Verification items for the finished model (mm, model axes). Face numbers are marked on the shaded views. Give positions to 0.01 mm unless a question says otherwise; leave off trailing zeros. Order: outer loops, then holes, each group sorted by start corner. A loop starts at its lowest first (then second) coordinate and runs counter-clockwise, first axis right, second up. Notation, with made-up numbers: (34.5, 59.25) - (47.5, 59.25) arc R27 cw to (47.5, 87.25) - close; hole circle Ø1 at (-0.5, 12). An arc over 180 degrees is marked (long way). Answer as a JSON object with one key per item and string values. Group by question number.
(1) Mould release check, pull along X, two halves, no side actions. Record for the marked faces 1, 2 and 3: +X half, -X half, draft (parallel to the pull), parting line (faces both ways), or undercut.
(2) Thickness scan on line 1 (X direction, y = 18, z = -4); line 2 (Y direction, x = 8.25, z = -1.5); line 3 (Z direction, x = 13, y = 52.5). Record the ranges inside material, lowest first.
(3) Section check B-B (x = 4). Record the boundary of the cut face in (y, z).
(4) Section check A-A (z = -4). Record the boundary of the cut face in (x, y).
(5) Depth check by flat-ended pin: pin 1 Ø12 at (x, y) = (11, 56.5) entering from +Z; pin 2 Ø10 at (x, y) = (4, 55.5) entering from -Z; pin 3 Ø5 at (x, z) = (26, -4) entering from +Y; pin 4 Ø3.5 at (x, z) = (4, -26) entering from -Y. Enter the tip coordinate at first touch or a pass-through.
(6) Section check C-C (y = 9). Record the boundary of the cut face in (x, z), then the cut area to 3 significant figures.
(7) Section check D-D (z = -15). Record the boundary of the cut face in (x, y), then the cut area to 3 significant figures.
```python
from build123d import *

# Parameters (mm, degrees)
IZIM1_W                     = 30
IZIM1_H                     = 30
Y_KSEKLIK_EKSTR_ZYON1_DEPTH = 40
IZIM2_R                     = 2
KES_EKSTR_ZYON1_DEPTH       = 40
IZIM3_R                     = 10
IZIM3_R_2                   = 4.25
Y_KSEKLIK_EKSTR_ZYON2_DEPTH = 40


with BuildPart() as part:
    # Çizim1 → Yükseklik-Ekstrüzyon1 (new body)
    with BuildSketch(Plane(origin=(0, 0, 0), x_dir=(1, 0, 0), z_dir=(0, 1, 0))):
        with Locations((15, 15)):
            Rectangle(IZIM1_W, IZIM1_H)
    extrude(amount=Y_KSEKLIK_EKSTR_ZYON1_DEPTH)

    # Çizim2 → Kes-Ekstrüzyon1 (cut)
    with BuildSketch(Plane(origin=(0, 40, 0), x_dir=(1, 0, 0), z_dir=(0, 1, 0))):
        with Locations(Location((4, 26, 0), (0, 0, 270))):
            Circle(IZIM2_R)
        with Locations(Location((26, 26, 0), (0, 0, 270))):
            Circle(IZIM2_R)
        with Locations(Location((26, 4, 0), (0, 0, 270))):
            Circle(IZIM2_R)
        with Locations(Location((4, 4, 0), (0, 0, 270))):
            Circle(IZIM2_R)
    extrude(amount=-KES_EKSTR_ZYON1_DEPTH, mode=Mode.SUBTRACT)

    # Çizim3 → Yükseklik-Ekstrüzyon2 (add)
    with BuildSketch(Plane(origin=(0, 40, 0), x_dir=(1, 0, 0), z_dir=(0, 1, 0))):
        with Locations(Location((15, 15, 0), (0, 0, 90))):
            Circle(IZIM3_R)
        with Locations(Location((15, 15, 0), (0, 0, 270))):
            Circle(IZIM3_R_2, mode=Mode.SUBTRACT)
    extrude(amount=Y_KSEKLIK_EKSTR_ZYON2_DEPTH)


solid = part.part
```
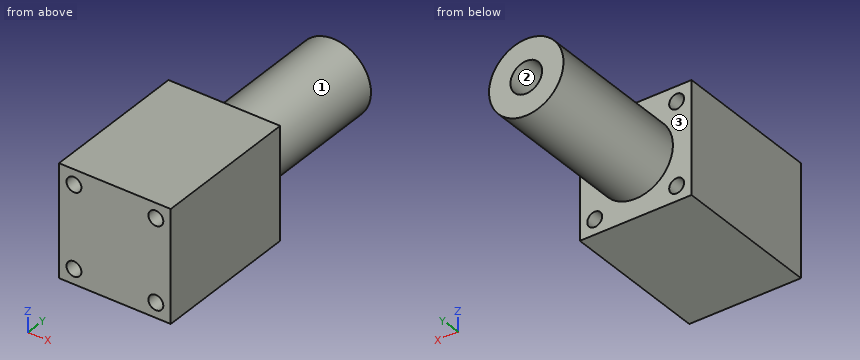
Solutions:
{
 "1": {"face 1": "parting line", "face 2": "undercut", "face 3": "draft"},
 "2": {"line 1": "x = 0 to 2, 6 to 24, 28 to 30", "line 2": "y = 0 to 40", "line 3": "z = -24.8 to -18.75, -11.25 to -5.2"},
 "3": {"outline": "(0, -30) - (40, -30) - (40, -28) - (0, -28) - close; (0, -24) - (40, -24) - (40, -6) - (0, -6) - close; (0, -2) - (40, -2) - (40, 0) - (0, 0) - close"},
 "4": {"outline": "(0, 0) - (2, 0) - (2, 40) - (0, 40) - close; (6, 0) - (24, 0) - (24, 40) - (6, 40) - close; (28, 0) - (30, 0) - (30, 40) - (28, 40) - close"},
 "5": {"pin 1": "stops at z = -5", "pin 2": "stops at z = -23", "pin 3": "stops at y = 40", "pin 4": "passes through"},
 "6": {"outline": "(0, -30) - (30, -30) - (30, 0) - (0, 0) - close; hole circle Ø4 at (4, -26); hole circle Ø4 at (4, -4); hole circle Ø4 at (26, -26); hole circle Ø4 at (26, -4)", "area": "850 mm2"},
 "7": {"outline": "(0, 0) - (30, 0) - (30, 40) - (25, 40) - (25, 80) - (19.25, 80) - (19.25, 40) - (10.75, 40) - (10.75, 80) - (5, 80) - (5, 40) - (0, 40) - close", "area": "1,660 mm2"}
}
